CAD build for the part. Positions are in the model's coordinates, mm. Face numbers are marked on the shaded views. A direction names the side the tool comes from. Round coordinates to 2 decimals unless told otherwise and drop trailing zeros. Return JSON: item names as keys, results as strings. Group by question number.
Q1. Which spindle directions (+Z, -Z, +X, -X, +Y, -Y) get a long thin tool onto all of the face, cutting with end or side? Do the marked faces 4 and 5. Say none if no direction does.
Q2. Probe line 1 along X through (y, z) = (-13, 41); line 2 along Y through (x, z) = (-4.5, 8); line 3 along X through (y, z) = (7, 38.5). List the from-to ranges inside material, lowest first.
Q3. Mould opens along Z. For the marked faces 1, 2 and 3 say: +Z half, -Z half, draft (parallel to the pull), parting line (faces both ways), or undercut.
Q4. Flat gauge pins, fed straight in: pin 1 (4 mm diameter, centred on x = -26.5, y = -17, fed in from +Z); pin 2 (4 mm diameter, centred on x = 16.5, z = 11, fed in from -Y); pin 3 (3 mm diameter, centred on x = -2, z = 21, fed in from -Y). Where does each tip first touch, or does it go through?
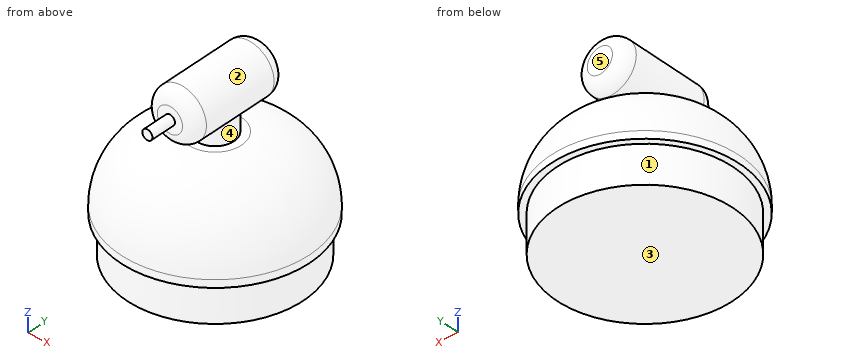
Autodesk Inventor part; units mm, degrees
ref_plane "YZ Plane" through (0, 0, 0) normal (1, 0, 0) x (0, 1, 0)
ref_plane "XZ Plane" through (0, 0, 0) normal (0, 1, 0) x (-1, 0, 0)
ref_plane "XY Plane" through (0, 0, 0) normal (0, 0, 1) x (1, 0, 0)
sketch "Sketch1" plane through (0, 0, 0) normal (0, 0, 1) x (1, 0, 0)
  circle A0 centre (0, 0) radius 37.5
  dimension "d0" = 75
extrude "Extrusion1" add sketch "Sketch1" along normal blind 30
sketch "Sketch2" plane through (0, 0, 30) normal (0, 0, 1) x (1, 0, 0)
  circle A0 centre (0, 0) radius 7.5
  dimension "d3" = 15
extrude "Extrusion2" add sketch "Sketch2" along normal blind 20
fillet "Fillet1" radius 27 1 edges at (-37.5, 0, 30)
sketch "Sketch3" plane through (0, 0, 0) normal (0, 0, -1) x (-1, 0, 0)
  circle A0 centre (0, 0) radius 35
  dimension "d7" = 70
extrude "Extrusion3" add sketch "Sketch3" along normal blind 15
sketch "Sketch7" plane through (0, 0, 0) normal (0, 1, 0) x (-1, 0, 0)
  circle A0 centre (0, 45) radius 10
  point P0 (0, 0)
  dimension "d22" = 20
extrude "Extrusion7" add sketch "Sketch7" along normal mid plane 40
sketch "Sketch8" plane through (0, -20, 45) normal (0, -1, 0) x (1, 0, 0)
  circle A0 centre (0, 0) radius 10
  circle A1 centre (0, 0) radius 2
  point P0 (0, -45)
  dimension "d25" = 4
extrude "Extrusion8" add sketch "Sketch8" along normal blind 10 contours A1
fillet "Fillet3" radius 5 2 edges at (10, 20, 45) (10, -20, 45)
properties part number "tapa gas"
Solution:
{
 "1": {"face 4": "none", "face 5": "+Z, +X, -X, +Y"},
 "2": {"line 1": "x = -9.17 to 9.17", "line 2": "y = -36.76 to 36.76", "line 3": "x = -7.6 to 7.6"},
 "3": {"face 1": "draft", "face 2": "undercut", "face 3": "-Z half"},
 "4": {"pin 1": "stops at z = 22.2", "pin 2": "stops at y = -33.46", "pin 3": "stops at y = -31.81"}
}
